Source: CAD feature listing. Evaluate the final solid. Frame: model axes, mm. A direction names the side the tool comes from. Give positions to 0.01 mm unless a question says otherwise; leave off trailing zeros. Order: outer loops, then holes, each group sorted by start corner. A loop starts at its lowest first (then second) coordinate and runs counter-clockwise, first axis right, second up. Notation, with made-up numbers: M -24,22.5 L 20,22.5 A22 cw 20,52.5 Z; hole C 41.25,57.25 d6. An arc over 180 degrees is marked long. Use CSV: the item, a comma, the result in double quotes. Start each with the question number.
1. Section query B-B, the plane x = 20.5. State how many separate pieces and enclosed holes the cut face has, plus the area to 3 significant figures.
2. Section query A-A, the plane y = 168. Return the cut outline in (x, z), plus the area to 3 significant figures.
3. Reachability of faces 4 (the cylindrical face through (14.65, 82.26, 75.08)), 5 (the cylindrical face through (1.972, 190.034, 73.521)), 6 (the flat face through (18, 162, 59)), 7 (the cylindrical face through (10.834, 8.822, 91.278)) from +Z, -Z, +X, -X, +Y, -Y: full face, straight path, thin tool, end or side. Return the list, or none.
4. Line query: line 1 along Z through (x, y) = (7.5, 147.7); line 2 along Y through (x, z) = (6, 70); line 3 along Z through (x, y) = (19.5, 81.4). Output: solid intervals per line, ascending. Write a range as [from, to].
5. Section query C-C, the plane z = 97.5. Return the cut outline in (x, y), plus the area to 3 significant figures.
6. Mould query, pull axis Z, two halves, no side actions, for faces 1 (the flat face through (13, 101, 120)), 2 (the cylindrical face through (14.647, 195.996, 74.038)), 3 (the flat face through (0, 99, 59)). Classes: released by +Z, released by -Z, zero draft, split by the parting line, or undercut.
7. Pin query (flat end, axial travel): P1, Ø4, axis at y = 167.5, z = 48.5, coming from the -X side; P2, Ø3.5, axis at y = 194, z = 73, coming from the +X side. Return the tip coordinate at first contact, or that it passes through.
from build123d import *

# Parameters (mm, degrees)
BOSS_EXTRUDE1_DEPTH            = 120
CBORE_FOR_M4_SHCS4_D           = 4.5
CBORE_FOR_M4_SHCS4_CBORE_D     = 8
CBORE_FOR_M4_SHCS4_CBORE_DEPTH = 4
M4_TAPPED_HOLE1_D              = 3.3
M5_TAPPED_HOLE1_D              = 4.2
M5_TAPPED_HOLE1_DEPTH          = 17.4
M5_TAPPED_HOLE1_TIP            = 1.2618073


with BuildPart() as part:
    # Sketch1 → Boss-Extrude1 (new body)
    with BuildSketch(Plane.XY):
        Polygon((0, 0), (0, 200), (25, 200), (25, 162), (11, 162), (11, 112), (25, 112), (25, 0), align=None)
    extrude(amount=BOSS_EXTRUDE1_DEPTH)

    # CBORE for M4 SHCS4 (through all)
    with Locations(Plane(origin=(0, 194, 73), x_dir=(0, 0, -1), z_dir=(-1, 0, 0))):
        with Locations((0, 0), (0, 26), (3, 46.3), (3, 66.3), (0, 86.6), (0, 112.6), (26, 112.6), (26, 86.6), (23, 66.3), (23, 46.3), (26, 26), (26, 0)):
            CounterBoreHole(CBORE_FOR_M4_SHCS4_D / 2, CBORE_FOR_M4_SHCS4_CBORE_D / 2, CBORE_FOR_M4_SHCS4_CBORE_DEPTH)

    # M4 Tapped Hole1 (through all)
    with Locations(Plane(origin=(0, 190, 16.7), x_dir=(0, 0, -1), z_dir=(-1, 0, 0))):
        with Locations((0, 0), (0, 60), (0, 120), (0, 180), (-86.6, 180), (-86.6, 120), (-86.6, 60), (-86.6, 0)):
            Hole(M4_TAPPED_HOLE1_D / 2)

    # M5 Tapped Hole1
    with Locations(Plane(origin=(12.5, 0, 90), x_dir=(-1, 0, 0), z_dir=(0, -1, 0))):
        with Locations((0, 0), (0, 30), (0, 60)):
            Hole(M5_TAPPED_HOLE1_D / 2, depth=M5_TAPPED_HOLE1_DEPTH)
            with Locations((0, 0, -(M5_TAPPED_HOLE1_DEPTH + M5_TAPPED_HOLE1_TIP / 2))):  # 118° drill point
                Cone(0, M5_TAPPED_HOLE1_D / 2, M5_TAPPED_HOLE1_TIP, mode=Mode.SUBTRACT)


solid = part.part
Result set:
1,separate pieces,"2"
1,enclosed holes,"14"
1,area,"17,800 mm2"
2,outline,"M 0,0 L 25,0 L 25,44.75 L 4,44.75 L 4,43 L 0,43 Z; M 0,51 L 4,51 L 4,49.25 L 25,49.25 L 25,70.75 L 4,70.75 L 4,69 L 0,69 Z; M 0,77 L 4,77 L 4,75.25 L 25,75.25 L 25,120 L 0,120 Z"
2,area,"2,750 mm2"
3,face 4,"+X, -X"
3,face 5,"-X"
3,face 6,"+Z, -Z, +X"
3,face 7,"-Y"
4,line 1,"[0, 47.75], [52.25, 67.75], [72.25, 120]"
4,line 2,"[0, 125.45], [129.95, 145.45], [149.95, 200]"
4,line 3,"[0, 44.75], [49.25, 70.75], [75.25, 120]"
5,outline,"M 0,0 L 25,0 L 25,112 L 11,112 L 11,162 L 25,162 L 25,200 L 0,200 Z"
5,area,"4,300 mm2"
6,face 1,"released by +Z"
6,face 2,"undercut"
6,face 3,"zero draft"
7,P1,"x = 4"
7,P2,"through"
